```python
from build123d import *

# Parameters (mm, degrees)
SKETCH1_R                                       = 9
BOSS_EXTRUDE1_DEPTH                             = 7.9
SKETCH2_R                                       = 3
CUT_EXTRUDE1_DEPTH                              = 3.1
SKETCH3_R                                       = 3.5
BOSS_EXTRUDE2_DEPTH                             = 4
TAPPED_HOLE_FOR_M2_5X0_45_HELICOIL1_D           = 2.55
TAPPED_HOLE_FOR_M2_5X0_45_HELICOIL1_DEPTH       = 6.85
TAPPED_HOLE_FOR_M2_5X0_45_HELICOIL1_CSINK_D     = 3.195
TAPPED_HOLE_FOR_M2_5X0_45_HELICOIL1_CSINK_ANGLE = 90
TAPPED_HOLE_FOR_M2_5X0_45_HELICOIL1_TIP         = 0.766097289
CHAMFER1_SIZE                                   = 0.1


with BuildPart() as part:
    # Sketch1 → Boss-Extrude1 (new body)
    with BuildSketch(Plane(origin=(0, 0, 0), x_dir=(1, 0, 0), z_dir=(0, 1, 0))):
        Circle(SKETCH1_R)
    extrude(amount=BOSS_EXTRUDE1_DEPTH)

    # Sketch2 → Cut-Extrude1 (cut)
    with BuildSketch(Plane(origin=(0, 7.9, 0), x_dir=(1, 0, 0), z_dir=(0, 1, 0))):
        Circle(SKETCH2_R)
    extrude(amount=-CUT_EXTRUDE1_DEPTH, mode=Mode.SUBTRACT)

    # Sketch3 → Boss-Extrude2 (add)
    with BuildSketch(Plane.XZ):
        Circle(SKETCH3_R)
    extrude(amount=BOSS_EXTRUDE2_DEPTH)

    # Tapped Hole for M2.5x0.45 Helicoil1
    with Locations(Plane(origin=(0, -4, 0), x_dir=(-1, 0, 0), z_dir=(0, -1, 0))):
        with Locations((0, 0)):
            CounterSinkHole(TAPPED_HOLE_FOR_M2_5X0_45_HELICOIL1_D / 2, TAPPED_HOLE_FOR_M2_5X0_45_HELICOIL1_CSINK_D / 2, depth=TAPPED_HOLE_FOR_M2_5X0_45_HELICOIL1_DEPTH, counter_sink_angle=TAPPED_HOLE_FOR_M2_5X0_45_HELICOIL1_CSINK_ANGLE)
            with Locations((0, 0, -(TAPPED_HOLE_FOR_M2_5X0_45_HELICOIL1_DEPTH + TAPPED_HOLE_FOR_M2_5X0_45_HELICOIL1_TIP / 2))):  # 118° drill point
                Cone(0, TAPPED_HOLE_FOR_M2_5X0_45_HELICOIL1_D / 2, TAPPED_HOLE_FOR_M2_5X0_45_HELICOIL1_TIP, mode=Mode.SUBTRACT)

    # Chamfer1
    chamfer1_edges = [part.edges().sort_by_distance(p)[0] for p in [
        (-3, 7.9, 0),
    ]]
    chamfer(chamfer1_edges, length=CHAMFER1_SIZE)


solid = part.part
```
Geometry: final body of the model. Coordinates: model frame, mm. A direction names the side the tool comes from. Round coordinates to 2 decimals unless told otherwise and drop trailing zeros. Write each loop counter-clockwise with the first axis right and the second up, starting at its lowest first coordinate (ties: lowest second). Pieces come first, ordered by that corner, then holes. Notation, with made-up numbers: (47, -29.75) -> (87, -29.75) arc R20 ccw to (87, -7.75) -> close; hole circle Ø7 at (89, 41). An arc over 180 degrees is marked (long way). Use CSV: the item, a comma, the result in double quotes. Start each with the question number.
Q1. Reachability of faces 1 (the face through (1, -4, -2)), 2 (the face through (3.233, -1.972, -1.341)), 3 (the face through (0, 4.8, 0)) from +Z, -Z, +X, -X, +Y, -Y: full face, straight path, thin tool, end or side. Return the list, or none.
Q2. Line query: L1, parallel to Z at x = 0, y = 6.25; L2, parallel to Z at x = 0, y = -2 (3 decimals). Output: solid intervals per line, ascending.
Q3. Section B-B (y = 4). Return loops of the section in (x, z), plus the area to 3 significant figures.
Q4. Section C-C (z = 6.5). Return loops of the section in (x, y), plus the area to 3 significant figures.
Q5. First-contact query: pin 1 Ø6.5 at (x, z) = (-0.5, 1) entering from +Y; pin 2 Ø1.5 at (x, y) = (2, 5) entering from +Z; pin 3 Ø5.5 at (x, z) = (0, 0) entering from +Y. Flat tips, straight axial feed; report the tip coordinate or a pass-through.
Q6. Section A-A (y = 5.75). Return loops of the section in (x, z).
Q7. Pull-direction query (Z, two-part tool) for faces 4 (the face through (-1.172, 3.895, -8.923)), 5 (the face through (-3, 6, 0)), 6 (the face through (0, 7.9, 4)); classes: pulls with the +Z half, pulls with the -Z half, needs draft (parallel to the pull), parting line crosses it, or undercut.
Q8. Section D-D (y = -2.5). Return loops of the section in (x, z) (3 decimals), plus the area to 3 significant figures.
Result sheet:
1,face 1,"+Z, -Z, +X, -X, -Y"
1,face 2,"-Y"
1,face 3,"+Y"
2,L1,"-9 to -3, 3 to 9"
2,L2,"-3.5 to -1.275, 1.275 to 3.5"
3,outline,"circle Ø18 at (0, 0)"
3,area,"254 mm²"
4,outline,"(-6.22, 0) -> (6.22, 0) -> (6.22, 7.9) -> (-6.22, 7.9) -> close"
4,area,"98.4 mm²"
5,pin 1,"y = 7.9"
5,pin 2,"z = 8.91"
5,pin 3,"y = 4.8"
6,outline,"circle Ø18 at (0, 0); hole circle Ø6 at (0, 0)"
7,face 4,"parting line crosses it"
7,face 5,"undercut"
7,face 6,"needs draft"
8,outline,"circle Ø7 at (0, 0); hole circle Ø2.55 at (0, 0)"
8,area,"33.4 mm²"
